```python
from build123d import *

# Parameters (mm, degrees)
F1_DEPTH = 63.5
F2_DEPTH = 25.4
F3_DEPTH = 7.9375
F4_DEPTH = 25.4
F0_W     = 25.4
F0_H     = 4.7498
F0_H_2   = 4.7752
F6_R     = 6.35


with BuildPart() as f1:
    # F0 (on Front) → F1 (new body, symmetric)
    with BuildSketch(Plane.XZ):
        Polygon((22.225, 9.525), (-41.275, 9.525), (-41.275, -9.525), (41.275, -9.525), (41.275, 9.525), align=None)
    extrude(amount=F1_DEPTH, both=True)

    # F0 (on Front) → F2 (join, symmetric)
    with BuildSketch(Plane.XZ):
        with BuildLine():
            Line((22.225, 27.0233751515), (22.225, 9.525))
            Line((22.225, 9.525), (41.275, 9.525))
            Line((41.275, 9.525), (41.275, 27.0233751515))
            ThreePointArc((41.275, 27.0233751515), (46.232053506, 38.5478738111), (58.0074811786, 42.8752))
            Line((58.0074811786, 42.8752), (60.325, 42.8752))
            Line((60.325, 42.8752), (60.325, 61.9252))
            Line((60.325, 61.9252), (58.4221034718, 61.9252))
            add(Edge.make_bspline(
                [(53.9455429382, 61.8010559243), (55.4372337649, 61.858340914), (56.9298403376, 61.8995627303), (58.4221034718, 61.9252)],
                knots=[108.7173325618, 108.7173325618, 108.7173325618, 108.7173325618, 112.6290078119, 112.6290078119, 112.6290078119, 112.6290078119], degree=3))
            ThreePointArc((53.9455429382, 61.8010559243), (31.3462087293, 50.5588798425), (22.225, 27.0233751515))
        make_face()
    extrude(amount=F2_DEPTH, both=True)

    # F0 (on Front) → F3 (join, symmetric)
    with BuildSketch(Plane.XZ):
        with BuildLine():
            add(Edge.make_bspline(
                [(-41.275, 9.525), (-28.2643212455, 46.2087638667), (12.486925514, 60.2089321217), (53.9455429382, 61.8010559243)],
                knots=[0, 0, 0, 0, 108.7173325618, 108.7173325618, 108.7173325618, 108.7173325618], degree=3))
            Line((-41.275, 9.525), (22.225, 9.525))
            Line((22.225, 9.525), (22.225, 27.0233751515))
            ThreePointArc((22.225, 27.0233751515), (31.3462087293, 50.5588798425), (53.9455429382, 61.8010559243))
        make_face()
    extrude(amount=F3_DEPTH, both=True)

    # F4 (add): a face of the model
    f4_faces = [f1.faces().sort_by_distance(p)[0] for p in [
        (60.325, 0, 52.4002),
    ]]
    extrude(f4_faces, amount=F4_DEPTH)

    # F0 (on Front) → F5 (revolve)
    with BuildSketch(Plane.XZ):
        with Locations((98.425, 64.3001)):
            Rectangle(F0_W, F0_H)
        Polygon((111.125, 61.9252), (85.725, 61.9252), (85.725, 52.3875), (85.725, 42.8752), (111.125, 42.8752), align=None)
        with Locations((98.425, 40.4876)):
            Rectangle(F0_W, F0_H_2)
    revolve(axis=Axis((85.725, 0, 52.3875), (0, 0, 1)))

    # F6
    f6_edges = [f1.edges().sort_by_distance(p)[0] for p in [
        (41.275, -63.5, 0),
        (-41.275, -63.5, 0),
        (41.275, 63.5, 0),
        (-41.275, 63.5, 0),
    ]]
    fillet(f6_edges, radius=F6_R)


solid = f1.part
```
Here's how the part is built. I have some questions about the finished solid (model axes, mm). A direction names the side the tool comes from. Coordinates: 2 decimals unless noted, no trailing zeros. Order: outer loops, then holes, each group sorted by start corner. A loop starts at its lowest first (then second) coordinate and runs counter-clockwise, first axis right, second up. Notation, with made-up numbers: (23.25, 46) - (50.25, 46) arc R8 cw to (50.25, 55) - close; hole circle Ø8 at (41.25, -2.5). An arc over 180 degrees is marked (long way). One line per question, with ' | ' between items. Start each with the question number.
1. Please list where these lines run through material, in increasing order: line 1 along Z through (x, y) = (-7, 48) (3 decimals); line 2 along Z through (x, y) = (60.5, 5); line 3 along Y through (x, z) = (6, 23). Write a range as [from, to].
2. If we section it at B-B (y = -34.5): Write out the boundary of the cut face in (x, z) (3 decimals), and give its area (3 significant figures).
3. I'm going to push flat-ended pins straight in: pin 1 Ø4 at (y, z) = (14.5, 27.5) entering from +X; pin 2 Ø8.5 at (x, y) = (72, -9.5) entering from -Z; pin 3 Ø12 at (x, z) = (66, 47) entering from +Y; pin 4 Ø6 at (x, z) = (-24, 43) entering from +Y. Where does each tip first touch, or does it pass through?
4. Which directions (+Z, -Z, +X, -X, +Y, -Y) give clear straight access to the entire face, cutting with the end or side of a thin tool? Please do faces 1 (the flat face through (-4, -7.938, 30)), 2 (the flat face through (60, 0, 61.925)), 3 (the flat face through (22.225, 17, 18)), 4 (the flat face through (86, 0, 38.1)), 5 (the cylindrical face through (46.1, -0.36, 38.42)).
5. If we section it at A-A (z = 6.5): Write out the boundary of the cut face in (x, y) (3 decimals).
Model answer:
1) line 1: z = [-9.525, 9.525] | line 2: z = [42.88, 61.93] | line 3: y = [-7.94, 7.94]
2) outline: (-41.275, -9.525) - (41.275, -9.525) - (41.275, 9.525) - (-41.275, 9.525) - close | area: 1,570 mm²
3) pin 1: stops at x = 41.47 | pin 2: stops at z = 38.1 | pin 3: stops at y = 25.4 | pin 4: passes through
4) face 1: +Z, -X, -Y | face 2: +Z, -X | face 3: +Z, -X, +Y | face 4: -Z, +X, +Y, -Y | face 5: -Z, +Y, -Y
5) outline: (-41.275, -57.15) arc R6.35 ccw to (-34.925, -63.5) - (34.925, -63.5) arc R6.35 ccw to (41.275, -57.15) - (41.275, 57.15) arc R6.35 ccw to (34.925, 63.5) - (-34.925, 63.5) arc R6.35 ccw to (-41.275, 57.15) - close
